The model under review builds one solid part; all positions refer to its coordinate system, in mm. Give positions to 0.01 mm unless a question says otherwise; leave off trailing zeros. Loops run counter-clockwise (first coordinate to the right, second up) from the corner with the lowest first, then second, coordinate; pieces in that order, holes last. Notation, with made-up numbers: M 37,15.5 L 59,15.5 A19 cw 59,33.5 Z; hole C 34.5,-28.75 d3. An arc over 180 degrees is marked long. Return JSON: item names as keys, results as strings. Group by question number.
```python
from build123d import *

# Parameters (mm, degrees)
SKETCH_W     = 93
SKETCH_H     = 42.5
SKETCH_R     = 11
PAD_DEPTH    = 7
SKETCH001_R  = 4
POCKET_DEPTH = 7.001


with BuildPart() as part:
    # Sketch → Pad (new body)
    with BuildSketch(Plane.XY):
        Rectangle(SKETCH_W, SKETCH_H)
        with Locations((29.5, 0)):
            Circle(SKETCH_R, mode=Mode.SUBTRACT)
        with Locations((-29.5, 0)):
            Circle(SKETCH_R, mode=Mode.SUBTRACT)
    extrude(amount=PAD_DEPTH)

    # Sketch001 → Pocket (cut, through all)
    with BuildSketch(Plane.XY.offset(7)):
        Circle(SKETCH001_R)
    extrude(amount=-POCKET_DEPTH, mode=Mode.SUBTRACT)


solid = part.part
```
(1) Add section D-D (x = -29.5). Write out the cut boundary in (y, z).
(2) Mouldability with a two-part tool opening along Y and no side actions: class faces 1 (the flat face through (-1, 21.25, 3)), 2 (the flat face through (-1, 5, 7)), 3 (the cylindrical face through (-0.867, -3.905, 3.549)) as released by +Y, released by -Y, zero draft, split by the parting line, or undercut.
(3) Add section A-A (y = 0). Write out the cut boundary in (x, z).
(4) Add section C-C (z = 1). Write out the cut boundary in (x, y).
(5) For probe 1 along Y at (x, z) = (-29.5, 3.75); probe 2 along X at (y, z) = (-7.5, 2); probe 3 along Y at (x, z) = (0, 2.5), list the stretches that pass through material, from the lowest coordinate up.
(6) Add section B-B (x = 0). Write out the cut boundary in (y, z).
Verdict:
{
 "1": {"outline": "M -21.25,0 L -11,0 L -11,7 L -21.25,7 Z; M 11,0 L 21.25,0 L 21.25,7 L 11,7 Z"},
 "2": {"face 1": "released by +Y", "face 2": "zero draft", "face 3": "undercut"},
 "3": {"outline": "M -46.5,0 L -40.5,0 L -40.5,7 L -46.5,7 Z; M -18.5,0 L -4,0 L -4,7 L -18.5,7 Z; M 4,0 L 18.5,0 L 18.5,7 L 4,7 Z; M 40.5,0 L 46.5,0 L 46.5,7 L 40.5,7 Z"},
 "4": {"outline": "M -46.5,-21.25 L 46.5,-21.25 L 46.5,21.25 L -46.5,21.25 Z; hole C -29.5,0 d22; hole C 0,0 d8; hole C 29.5,0 d22"},
 "5": {"probe 1": "y = -21.25 to -11, 11 to 21.25", "probe 2": "x = -46.5 to -37.55, -21.45 to 21.45, 37.55 to 46.5", "probe 3": "y = -21.25 to -4, 4 to 21.25"},
 "6": {"outline": "M -21.25,0 L -4,0 L -4,7 L -21.25,7 Z; M 4,0 L 21.25,0 L 21.25,7 L 4,7 Z"}
}
